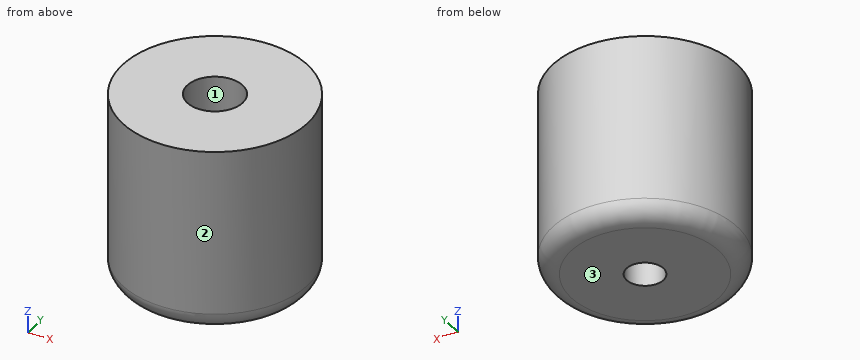
```python
from build123d import *

# Parameters (mm, degrees)
ESQUISSE1_R             = 5
BOSS_EXTRU_1_DEPTH      = 10
ESQUISSE2_R             = 1.5
ENL_V_MAT_EXTRU_1_DEPTH = 7
ESQUISSE3_R             = 1
ENL_V_MAT_EXTRU_2_DEPTH = 7
CONG_1_R                = 1


with BuildPart() as part:
    # Esquisse1 → Boss.-Extru.1 (new body)
    with BuildSketch(Plane.XY):
        Circle(ESQUISSE1_R)
    extrude(amount=BOSS_EXTRU_1_DEPTH)

    # Esquisse2 → Enlèv. mat.-Extru.1 (cut)
    with BuildSketch(Plane.XY.offset(10)):
        Circle(ESQUISSE2_R)
    extrude(amount=-ENL_V_MAT_EXTRU_1_DEPTH, mode=Mode.SUBTRACT)

    # Esquisse3 → Enlèv. mat.-Extru.2 (cut)
    with BuildSketch(Plane.XY.offset(3)):
        Circle(ESQUISSE3_R)
    extrude(amount=-ENL_V_MAT_EXTRU_2_DEPTH, mode=Mode.SUBTRACT)

    # Congé1
    cong_1_edges = [part.edges().sort_by_distance(p)[0] for p in [
        (-5, 0, 0),
    ]]
    fillet(cong_1_edges, radius=CONG_1_R)


solid = part.part
```
Model file for the job. Use its own axes, mm. Face numbers are marked on the shaded views. Give positions to 0.01 mm unless a question says otherwise; leave off trailing zeros. Loops run counter-clockwise (first coordinate to the right, second up) from the corner with the lowest first, then second, coordinate; pieces in that order, holes last. Notation, with made-up numbers: (39.5, 88) -> (90.5, 88) arc R18 ccw to (90.5, 100) -> close; hole circle Ø1 at (-32, 20). An arc over 180 degrees is marked (long way). Write each question's results on one line, items separated by ' | '.
(1) Flat gauge pins, fed straight in: pin 1 Ø5 at (x, z) = (3, 6) entering from +Y; pin 2 Ø1 at (x, z) = (3.5, 6.5) entering from -Y. Where does each tip first touch, or does it go through?
Geometry results:
pin 1: stops at y = 4.97 | pin 2: stops at y = -4
(2) Probe line 1 along Y through (x, z) = (0, 8.25); line 2 along Y through (x, z) = (0, 2.15); line 3 along Z through (x, y) = (-0.25, -1). List the from-to ranges inside material, lowest first.
Geometry results:
line 1: y = -5 to -1.5, 1.5 to 5 | line 2: y = -5 to -1, 1 to 5 | line 3: z = 0 to 3
(3) Cut at D-D on z = 1.5. List the corners of the cut face in (x, y), and give its area (3 significant figures).
Geometry results:
outline: circle Ø10 at (0, 0); hole circle Ø2 at (0, 0) | area: 75.4 mm²
(4) Cut at C-C on z = 8. List the corners of the cut face in (x, y).
Geometry results:
outline: circle Ø10 at (0, 0); hole circle Ø3 at (0, 0)
(5) Pull direction X, two halves, no side cores. Call the marked faces 1, 2 and 3: released by +X, released by -X, zero draft, split by the parting line, or undercut.
Geometry results:
face 1: undercut | face 2: split by the parting line | face 3: zero draft
(6) Cut at A-A on y = 0. List the corners of the cut face in (x, z).
Geometry results:
outline: (-5, 1) arc R1 ccw to (-4, 0) -> (-1, 0) -> (-1, 3) -> (-1.5, 3) -> (-1.5, 10) -> (-5, 10) -> close; (1, 0) -> (4, 0) arc R1 ccw to (5, 1) -> (5, 10) -> (1.5, 10) -> (1.5, 3) -> (1, 3) -> close
